Verification items for the finished model (mm, model axes). Face numbers are marked on the shaded views. A direction names the side the tool comes from. Give positions to 0.01 mm unless a question says otherwise; leave off trailing zeros. Loops run counter-clockwise (first coordinate to the right, second up) from the corner with the lowest first, then second, coordinate; pieces in that order, holes last. Notation, with made-up numbers: M 32.5,-30 L 66.5,-30 A22 cw 66.5,-22 Z; hole C 20,44 d6. An arc over 180 degrees is marked long. Use CSV: the item, a comma, the result in double quotes.
from build123d import *

# Parameters (mm, degrees)
SKETCH_1_R            = 2.75
EXTRUDE_248_DEPTH     = 3
CUT_EXTRUDE_378_DEPTH = 1.3
SKETCH_3_R            = 1.5
EXTRUDE_479_DEPTH     = 32


with BuildPart() as part:
    # 草图1 → Extrude 248 (new body)
    with BuildSketch(Plane(origin=(0, 0, 0), x_dir=(1, 0, 0), z_dir=(0, 1, 0))):
        Circle(SKETCH_1_R)
    extrude(amount=EXTRUDE_248_DEPTH)

    # 草图2 → Cut-Extrude 378 (cut)
    with BuildSketch(Plane(origin=(0, 3, 0), x_dir=(1, 0, 0), z_dir=(0, 1, 0))):
        Polygon((1.443375673, 0), (0.721687836, 1.25), (-0.721687836, 1.25), (-1.443375673, 0), (-0.721687836, -1.25), (0.721687836, -1.25), align=None)
    extrude(amount=-CUT_EXTRUDE_378_DEPTH, mode=Mode.SUBTRACT)

    # 草图3 → Extrude 479 (add)
    with BuildSketch(Plane.XZ):
        Circle(SKETCH_3_R)
    extrude(amount=EXTRUDE_479_DEPTH)


solid = part.part
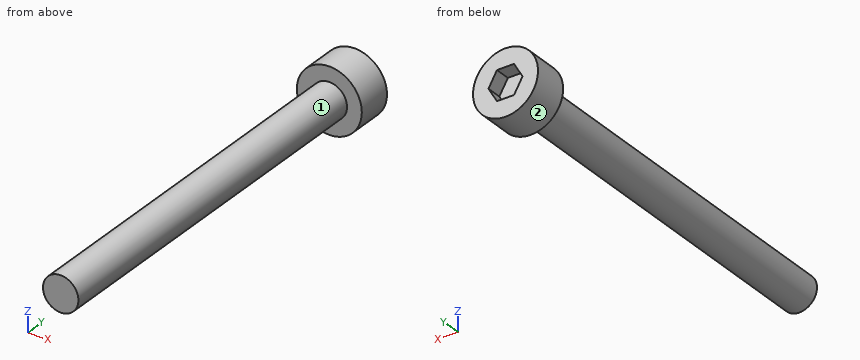
(1) Section check A-A on x = 0. Record the cut outline in (y, z), plus the area to 3 significant figures.
Calculated:
outline,"M -32,-1.5 L 0,-1.5 L 0,-2.75 L 3,-2.75 L 3,-1.25 L 1.7,-1.25 L 1.7,1.25 L 3,1.25 L 3,2.75 L 0,2.75 L 0,1.5 L -32,1.5 Z"
area,"109 mm²"
(2) Scan lines: L1, parallel to Y at x = 1.75, z = 1.6; L2, parallel to Y at x = 0.1, z = -1; L3, parallel to X at y = -9, z = 0.4. Record each from-to range of solid material in increasing order. Write a range as from..to.
Calculated:
L1,"y = 0..3"
L2,"y = -32..1.7"
L3,"x = -1.45..1.45"
(3) Depth check by flat-ended pin: pin 1 Ø0.6 at (x, y) = (0.5, 2.5) entering from -Z; pin 2 Ø1.5 at (y, z) = (-23.5, -1) entering from -X; pin 3 Ø3 at (x, y) = (-0.5, -20) entering from -Z. Enter the tip coordinate at first touch or a pass-through.
Calculated:
pin 1,"stops at z = -2.74"
pin 2,"stops at x = -1.48"
pin 3,"stops at z = -1.5"
(4) Section check B-B on z = 0.4. Record the cut outline in (x, y), plus the area to 3 significant figures.
Calculated:
outline,"M -2.72,0 L -1.45,0 L -1.45,-32 L 1.45,-32 L 1.45,0 L 2.72,0 L 2.72,3 L 1.21,3 L 1.21,1.7 L -1.21,1.7 L -1.21,3 L -2.72,3 Z"
area,"106 mm²"
(5) Section check D-D on z = 1.8. Record the cut outline in (x, y).
Calculated:
outline,"M -2.08,0 L 2.08,0 L 2.08,3 L -2.08,3 Z"
(6) Section check C-C on y = -3. Record the cut outline in (x, z).
Calculated:
outline,"C 0,0 d3"
(7) Tool access check on the marked faces 1 and 2. Record the directions out of +Z, -Z, +X, -X, +Y, -Y that give a thin tool (end or side, any length) a straight path to the whole face; none if there is none.
Calculated:
face 1,"-Y"
face 2,"+Y, -Y"
